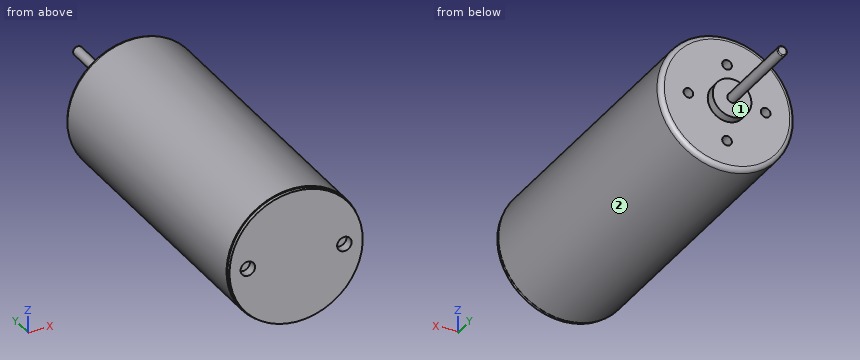
from build123d import *

# Parameters (mm, degrees)
ESBO_O1_R                = 3.5
RESSALTO_EXTRUS_O1_DEPTH = 16
ESBO_O2_R                = 3.45
RESSALTO_EXTRUS_O2_DEPTH = 0.2
ESBO_O3_R                = 0.375
CORTE_EXTRUS_O1_DEPTH    = 0.5
ESBO_O4_R                = 1
RESSALTO_EXTRUS_O3_DEPTH = 0.5
ESBO_O5_R                = 0.25
RESSALTO_EXTRUS_O4_DEPTH = 5
FILETE1_R                = 0.25
FILETE2_R                = 0.05
ESBO_O6_R                = 0.25
CORTE_EXTRUS_O2_DEPTH    = 1


with BuildPart() as part:
    # Esboço1 → Ressalto-extrusão1 (new body)
    with BuildSketch(Plane(origin=(0, 0, 0), x_dir=(1, 0, 0), z_dir=(0, 1, 0))):
        with Locations(Location((0, 0, 0), (0, 0, 270))):
            Circle(ESBO_O1_R)
    extrude(amount=RESSALTO_EXTRUS_O1_DEPTH)

    # Esboço2 → Ressalto-extrusão2 (add)
    with BuildSketch(Plane.XZ):
        with Locations(Location((0, 0, 0), (0, 0, 270))):
            Circle(ESBO_O2_R)
    extrude(amount=RESSALTO_EXTRUS_O2_DEPTH)

    # Esboço3 → Corte-extrusão1 (cut)
    with BuildSketch(Plane.XZ.offset(0.2)):
        with Locations(Location((-2.5, 0, 0), (0, 0, 270))):
            Circle(ESBO_O3_R)
        with Locations(Location((2.5, 0, 0), (0, 0, 270))):
            Circle(ESBO_O3_R)
    extrude(amount=-CORTE_EXTRUS_O1_DEPTH, mode=Mode.SUBTRACT)

    # Esboço4 → Ressalto-extrusão3 (add)
    with BuildSketch(Plane(origin=(0, 16, 0), x_dir=(1, 0, 0), z_dir=(0, 1, 0))):
        with Locations(Location((0, 0, 0), (0, 0, 270))):
            Circle(ESBO_O4_R)
    extrude(amount=RESSALTO_EXTRUS_O3_DEPTH)

    # Esboço5 → Ressalto-extrusão4 (add)
    with BuildSketch(Plane(origin=(0, 16.5, 0), x_dir=(1, 0, 0), z_dir=(0, 1, 0))):
        with Locations(Location((0, 0, 0), (0, 0, 270))):
            Circle(ESBO_O5_R)
    extrude(amount=RESSALTO_EXTRUS_O4_DEPTH)

    # Filete1
    filete1_edges = [part.edges().sort_by_distance(p)[0] for p in [
        (0, 16, -3.5),
    ]]
    fillet(filete1_edges, radius=FILETE1_R)

    # Filete2
    filete2_edges = [part.edges().sort_by_distance(p)[0] for p in [
        (0, 21.5, -0.25),
    ]]
    fillet(filete2_edges, radius=FILETE2_R)

    # Esboço6 → Corte-extrusão2 (cut)
    with BuildSketch(Plane(origin=(0, 16, 0), x_dir=(1, 0, 0), z_dir=(0, 1, 0))):
        with Locations(Location((0, 2, 0), (0, 0, 270))):
            Circle(ESBO_O6_R)
        with Locations(Location((2, 0, 0), (0, 0, 270))):
            Circle(ESBO_O6_R)
        with Locations(Location((0, -2, 0), (0, 0, 270))):
            Circle(ESBO_O6_R)
        with Locations(Location((-2, 0, 0), (0, 0, 270))):
            Circle(ESBO_O6_R)
    extrude(amount=-CORTE_EXTRUS_O2_DEPTH, mode=Mode.SUBTRACT)


solid = part.part
Can you work these out from the model? Positions are in its coordinate system, mm. Face numbers are marked on the shaded views. A direction names the side the tool comes from. Give positions to 0.01 mm unless a question says otherwise; leave off trailing zeros. Loops run counter-clockwise (first coordinate to the right, second up) from the corner with the lowest first, then second, coordinate; pieces in that order, holes last. Notation, with made-up numbers: M -4.75,-10.75 L 47.25,-10.75 A34 ccw 47.25,22.25 Z; hole C 22.5,-5 d2. An arc over 180 degrees is marked long. One line per item, written item: value. Start each with the question number.
1) On a 3-axis mill with a long thin cutter (end or side, diameter ignored), from which of +Z, -Z, +X, -X, +Y, -Y can I reach the whole of each face in a straight line? I mean the marked faces 1 and 2. Say none if no direction works.
2) If I drill on line 1 (X direction, y = 15.6, z = 0); line 2 (X direction, y = 0.25, z = 0) (3 decimals); line 3 (X direction, y = 15.7, z = 2), over which ranges is the centre line in solid material (lowest first)? Write a range as [from, to].
3) If we section it at B-B, the plane y = 1.5: Write out the boundary of the cut face in (x, z), and give its area (3 significant figures).
4) If we section it at A-A, the plane y = 20: Write out the boundary of the cut face in (x, z), and give its area (3 significant figures).
5) I'm going to push flat-ended pins straight in: pin 1 (0.6 mm diameter, centred on x = 0, z = -2, fed in from +Y); pin 2 (1 mm diameter, centred on x = -1, z = -0.5, fed in from +Y). Where does each tip first touch, or does it pass through?
Completed:
1. face 1: +Y
1. face 2: +Y, -Y
2. line 1: x = [-3.5, -2.25], [-1.75, 1.75], [2.25, 3.5]
2. line 2: x = [-3.5, -2.875], [-2.125, 2.125], [2.875, 3.5]
2. line 3: x = [-2.87, -0.25], [0.25, 2.87]
3. outline: C 0,0 d7
3. area: 38.5 mm^2
4. outline: C 0,0 d0.5
4. area: 0.196 mm^2
5. pin 1: stops at y = 16
5. pin 2: stops at y = 16.5
